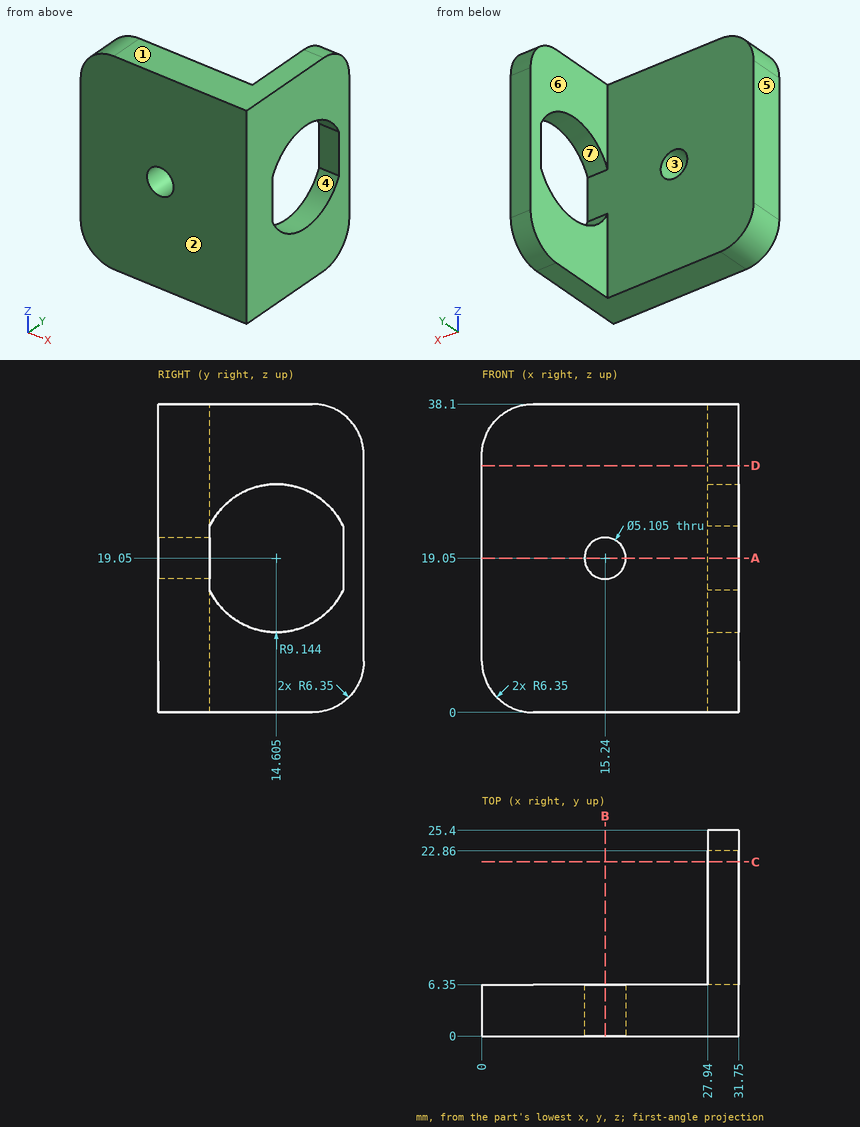
For this review, use the dimensioned drawing (mm, ordinates from the lowest corner) and the shaded views. A direction names the side the tool comes from. Give positions to 0.01 mm unless a question says otherwise; leave off trailing zeros. Order: outer loops, then holes, each group sorted by start corner. A loop starts at its lowest first (then second) coordinate and runs counter-clockwise, first axis right, second up. Notation, with made-up numbers: (9.25, -1.75) -> (17.25, -1.75) arc R11 cw to (17.25, 8.25) -> close; hole circle Ø10 at (7.5, 27.5). An arc over 180 degrees is marked (long way). Write item = value, one per line. Start each with the question number.
(1) Take a section at C-C (y = 21.5). Write out the cut boundary in (x, z).
(2) Tool access review of the marked faces 5, 6 and 7: name each direction out of +Z, -Z, +X, -X, +Y, -Y from which nothing blocks a thin tool from reaching the whole face with its end or side.
(3) Draft analysis for pull direction Z (two halves, no side actions). For the marked faces 1, 2, 3 and 4, state which applies: +Z half, -Z half, draft (parallel to the pull), parting line (faces both ways), or undercut.
(4) Take a section at B-B (x = 15.24). Write out the cut boundary in (y, z).
(5) Take a section at D-D (z = 30.5). Write out the cut boundary in (x, y).
(6) For L1, parallel to Z at x = 15.24, y = 4.25; L2, parallel to X at y = 12, z = 4.5; L3, parallel to Y at x = 16.5, z = 7, list the stretches that pass through material, from the lowest coordinate up. Write a range as from..to.
(7) Take a section at A-A (z = 19.05). Write out the cut boundary in (x, y), plus the area to 3 significant figures.
(8) For pin 1 Ø1.9 at (x, z) = (30, 17.5) entering from -Y; pin 2 Ø3 at (x, z) = (19.5, 14) entering from +Y; pin 3 Ø9.5 at (y, z) = (15.5, 20.5) entering from -X, all flat-tipped, find the tip position at first contact; note any pin that passes through.
Returned:
q1.outline = (27.94, 0.49) -> (31.75, 0.49) -> (31.75, 13.04) -> (27.94, 13.04) -> close; (27.94, 25.06) -> (31.75, 25.06) -> (31.75, 37.61) -> (27.94, 37.61) -> close
q2.face_5 = +Z, -Z, -X, +Y, -Y
q2.face_6 = +Z, -Z, -X, +Y
q2.face_7 = +X, -X
q3.face_1 = +Z half
q3.face_2 = draft
q3.face_3 = undercut
q3.face_4 = undercut
q4.outline = (0, 0) -> (6.35, 0) -> (6.35, 16.5) -> (0, 16.5) -> close; (0, 21.6) -> (6.35, 21.6) -> (6.35, 38.1) -> (0, 38.1) -> close
q5.outline = (0, 0) -> (31.75, 0) -> (31.75, 25.4) -> (27.94, 25.4) -> (27.94, 6.35) -> (0, 6.35) -> close
q6.L1 = 0..16.5, 21.6..38.1
q6.L2 = 27.94..31.75
q6.L3 = 0..6.35
q7.outline = (0, 0) -> (12.69, 0) -> (12.69, 6.35) -> (0, 6.35) -> close; (17.79, 0) -> (31.75, 0) -> (31.75, 6.35) -> (17.79, 6.35) -> close; (27.94, 22.86) -> (31.75, 22.86) -> (31.75, 25.4) -> (27.94, 25.4) -> close
q7.area = 179 mm²
q8.pin_1 = 0
q8.pin_2 = 6.35
q8.pin_3 = through
